Source: three-view drawing plus pictorial views. Frame: mm from the lowest corner of the part. Round coordinates to 2 decimals unless told otherwise and drop trailing zeros. Loops run counter-clockwise (first coordinate to the right, second up) from the corner with the lowest first, then second, coordinate; pieces in that order, holes last. Notation, with made-up numbers: (-29, -31) -> (7, -31) arc R23 cw to (7, -14) -> close; hole circle Ø11 at (3.25, -37). An arc over 180 degrees is marked (long way). Answer in a Markdown table with one row per item.
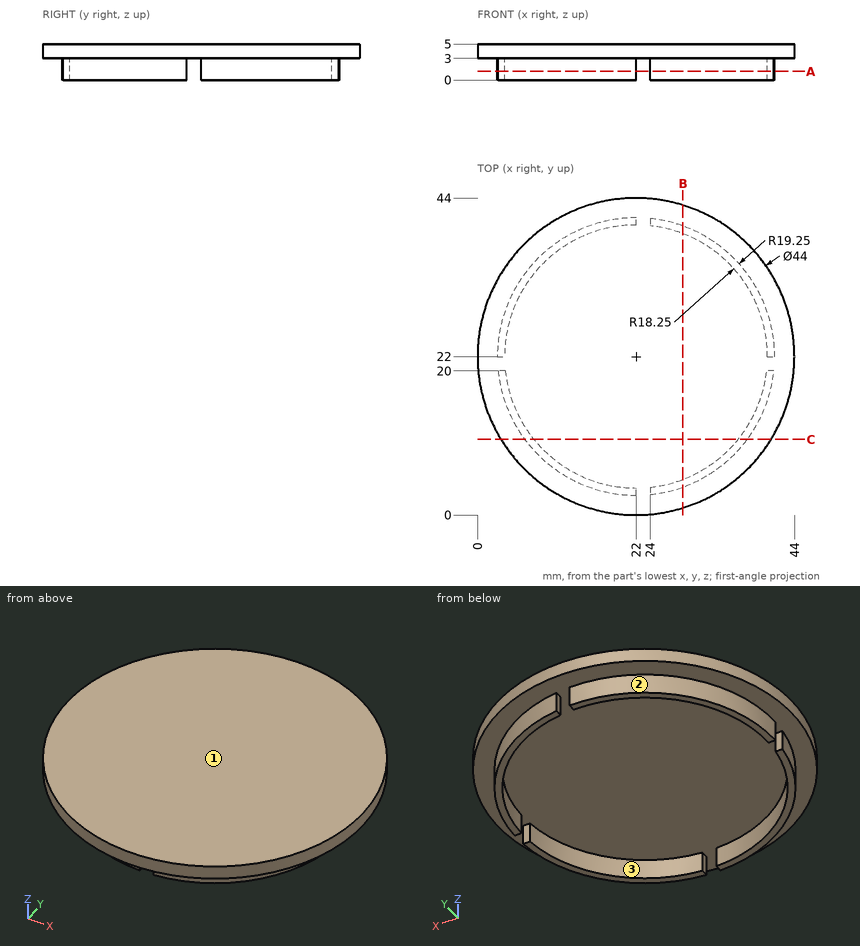
Item 1: Cut plane B-B (x = 28.5). Output: boundary loops of the cut face in (y, z), then the cut area to 3 significant figures.
Answer:
| item | result |
|---|---|
| outline | (0.98, 3) -> (3.88, 3) -> (3.88, 0) -> (4.95, 0) -> (4.95, 3) -> (39.05, 3) -> (39.05, 0) -> (40.12, 0) -> (40.12, 3) -> (43.02, 3) -> (43.02, 5) -> (0.98, 5) -> close |
| area | 90.5 mm² |
Item 2: Cut plane A-A (z = 1.2). Output: boundary loops of the cut face in (x, y).
Answer:
| item | result |
|---|---|
| outline | (2.75, 22) -> (3.75, 22) arc R18.25 cw to (22, 40.25) -> (22, 41.25) arc R19.25 ccw to start; (2.85, 20) arc R19.25 ccw to (22, 2.75) -> (22, 3.75) arc R18.25 cw to (3.86, 20) -> close; (24, 2.85) arc R19.25 ccw to (41.15, 20) -> (40.14, 20) arc R18.25 cw to (24, 3.86) -> close; (24, 40.14) arc R18.25 cw to (40.25, 22) -> (41.25, 22) arc R19.25 ccw to (24, 41.15) -> close |
Item 3: Line query: probe 1 along Z at (x, y) = (25, 27); probe 2 along Y at (x, z) = (12, 2.5); probe 3 along X at (y, z) = (10.5, 0.3). Output: solid intervals per line, ascending. Write a range as [from, to].
Answer:
| item | result |
|---|---|
| probe 1 | z = [3, 5] |
| probe 2 | y = [5.55, 6.73], [37.27, 38.45] |
| probe 3 | x = [6.56, 7.83], [36.17, 37.44] |
Item 4: Draft query along X for the marked faces 1, 2 and 3. Return one class per face: pulls with the +X half, pulls with the -X half, needs draft (parallel to the pull), parting line crosses it, or undercut.
Answer:
| item | result |
|---|---|
| face 1 | needs draft |
| face 2 | pulls with the -X half |
| face 3 | undercut |
Item 5: Pin query (flat end, axial travel): pin 1 Ø3 at (y, z) = (12.5, 0.5) entering from -X; pin 2 Ø4 at (x, y) = (27, 15.5) entering from -Z; pin 3 Ø1.5 at (y, z) = (16, 3) entering from +X. Return the tip coordinate at first contact, or that it passes through.
Answer:
| item | result |
|---|---|
| pin 1 | stops at x = 4.49 |
| pin 2 | stops at z = 3 |
| pin 3 | stops at x = 43.36 |
Item 6: Cut plane C-C (y = 10.5). Output: boundary loops of the cut face in (x, z) (3 decimals), then the cut area to 3 significant figures.
Answer:
| item | result |
|---|---|
| outline | (3.245, 3) -> (6.563, 3) -> (6.563, 0) -> (7.829, 0) -> (7.829, 3) -> (36.171, 3) -> (36.171, 0) -> (37.437, 0) -> (37.437, 3) -> (40.755, 3) -> (40.755, 5) -> (3.245, 5) -> close |
| area | 82.6 mm² |
